Here's how the part is built. I have some questions about the finished solid (model axes, mm). A direction names the side the tool comes from. Coordinates: 2 decimals unless noted, no trailing zeros. Loops run counter-clockwise (first coordinate to the right, second up) from the corner with the lowest first, then second, coordinate; pieces in that order, holes last. Notation, with made-up numbers: (14.5, 75) -> (46.5, 75) arc R11 ccw to (46.5, 91) -> close; hole circle Ø8 at (-1, 76.25). An arc over 180 degrees is marked (long way). Answer as a JSON object with one key per item and string values. Group by question number.
Q1. I want a section at C-C on y = -27. Write out the boundary of the cut face in (x, z), then the cut area to 3 significant figures.
Q2. I need wall thicknesses on line 1 (Y direction, x = -29, z = 10); line 2 (X direction, y = -6, z = 9); line 3 (Y direction, x = -20.5, z = 7.5). Which ranges of each line are inside material? Lowest first, please.
Q3. I want a section at A-A on z = 9.5. Count the separate pieces of the cut face and the enclosed holes in it, then the cut area to 3 significant figures.
Q4. I'm going to push flat-ended pins straight in: pin 1 (6 mm diameter, centred on x = -12, y = -9, fed in from -Z); pin 2 (8.5 mm diameter, centred on x = 16.84, y = 10.22, fed in from +Z). Where does each tip first touch, or does it pass through?
Q5. On a 3-axis mill with a long thin cutter (end or side, diameter ignored), from which of +Z, -Z, +X, -X, +Y, -Y can I reach the whole of each face in a straight line? I mean faces 1 (the flat face through (2, 39.573, 6)), 2 (the cylindrical face through (-32.5, 19.4, 9.6)). Say none if no direction works.
Q6. I want a section at D-D on x = -29. Write out the boundary of the cut face in (y, z), then the cut area to 3 significant figures.
Q7. I want a section at B-B on x = 0. Write out the boundary of the cut face in (y, z).
Q8. Thinking about a two-plate mould opening in X: for faces 3 (the flat face through (41.3, -8, 6)), 4 (the cylindrical face through (-30.02, -5.32, 9.57)), 5 (the flat face through (-1, -53.676, 6)), 6 (the flat face through (17, 10, 6.35)), which applies, released by +X, released by -X, zero draft, split by the parting line, or undercut?
```python
from build123d import *

# Parameters (mm, degrees)
F0_R     = 9.227752
F0_R_2   = 10.316944
F1_DEPTH = 12.7
F2_R     = 7.603738
F2_R_2   = 5.536052
F2_R_3   = 7.326338
F2_R_4   = 7.055645
F2_R_5   = 10.428743
F2_R_6   = 6.147535
F2_R_7   = 6.569287
F2_R_8   = 5.291244
F3_DEPTH = 6.35


with BuildPart() as f1:
    # F0 (on Top) → F1 (new body)
    with BuildSketch(Plane.XY):
        with BuildLine():
            Line((12.50172, 39.573293), (-25.80679, 39.573293))
            ThreePointArc((-25.80679, 39.573293), (-19.351501, 17.287133), (-42.451348, 15.109803))
            Line((-42.451348, 15.109803), (-42.451348, -53.675774))
            Line((-42.451348, -53.675774), (-26.046417, -53.675774))
            ThreePointArc((-26.046417, -53.675774), (-15.397607, -31.799477), (-4.748798, -53.675774))
            Line((-4.748798, -53.675774), (16.548831, -53.675774))
            Line((16.548831, -53.675774), (41.300125, -53.675774))
            Line((41.300125, -53.675774), (41.300125, -43.841226))
            ThreePointArc((41.300125, -43.841226), (32.662888, -31.226924), (41.300125, -18.612622))
            Line((41.300125, -18.612622), (41.300125, 39.573293))
            Line((41.300125, 39.573293), (31.532556, 39.573293))
            ThreePointArc((31.532556, 39.573293), (22.017138, 5.274796), (12.50172, 39.573293))
        make_face()
        with BuildLine():
            ThreePointArc((25.758617, -44.465989), (23.061133, -50.978291), (16.548831, -53.675774))
            ThreePointArc((16.548831, -53.675774), (10.036529, -37.953687), (25.758617, -44.465989))
        make_face(mode=Mode.SUBTRACT)
        with Locations((20.865915, -13.382968)):
            Circle(F0_R, mode=Mode.SUBTRACT)
        with Locations((-28.06106, -5.612212)):
            Circle(F0_R_2, mode=Mode.SUBTRACT)
        with BuildLine():
            Line((31.532556, 39.573293), (12.50172, 39.573293))
            ThreePointArc((12.50172, 39.573293), (22.017138, 5.274796), (31.532556, 39.573293))
        make_face()
        with BuildLine():
            Line((-25.80679, 39.573293), (-37.798287, 39.573293))
            ThreePointArc((-37.798287, 39.573293), (-40.274021, 38.209652), (-42.451348, 36.407427))
            Line((-42.451348, 36.407427), (-42.451348, 15.109803))
            ThreePointArc((-42.451348, 15.109803), (-19.351501, 17.287133), (-25.80679, 39.573293))
        make_face()
        with BuildLine():
            ThreePointArc((-4.748798, -53.675774), (-15.397607, -31.799477), (-26.046417, -53.675774))
            Line((-26.046417, -53.675774), (-4.748798, -53.675774))
        make_face()
        with Locations((-28.06106, -5.612212)):
            Circle(F0_R_2)
        with Locations((20.865915, -13.382968)):
            Circle(F0_R)
        with BuildLine():
            ThreePointArc((25.758617, -44.465989), (10.036529, -37.953687), (16.548831, -53.675774))
            ThreePointArc((16.548831, -53.675774), (23.061133, -50.978291), (25.758617, -44.465989))
        make_face()
        with BuildLine():
            Line((41.300125, -43.841226), (41.300125, -18.612622))
            ThreePointArc((41.300125, -18.612622), (32.662888, -31.226924), (41.300125, -43.841226))
        make_face()
    extrude(amount=F1_DEPTH)

    # F2 (on face) → F3 (cut)
    with BuildSketch(Plane.XY.offset(12.7)):
        with Locations((-26.909837, 14.246385)):
            Circle(F2_R)
        with Locations((31.802539, -24.895199)):
            Circle(F2_R_2)
        with Locations((-32.090344, -37.558652)):
            Circle(F2_R_3)
        with Locations((16.836636, 10.217104)):
            Circle(F2_R_4)
        with Locations((3.309769, -40.724512)):
            Circle(F2_R_5)
        with Locations((0, 26.046421)):
            Circle(F2_R_6)
        with Locations((-23.456169, -5.612212)):
            Circle(F2_R_7)
        with Locations((15.109802, -9.929299)):
            Circle(F2_R_8)
    extrude(amount=-F3_DEPTH, mode=Mode.SUBTRACT)


solid = f1.part
```
Result set:
{
 "1": {"outline": "(-42.45, 0) -> (41.3, 0) -> (41.3, 12.7) -> (36.92, 12.7) -> (36.92, 6.35) -> (26.68, 6.35) -> (26.68, 12.7) -> (-42.45, 12.7) -> close", "area": "999 mm²"},
 "2": {"line 1": "y = -53.68 to -44.2, -30.92 to -9.14, -2.09 to 6.94, 21.56 to 39.57", "line 2": "x = -42.45 to -30.01, -16.9 to 11.57, 18.65 to 41.3", "line 3": "y = -53.68 to -11.48, 0.25 to 10.16, 18.34 to 39.57"},
 "3": {"separate pieces": "1", "enclosed holes": "8", "area": "6,520 mm²"},
 "4": {"pin 1": "stops at z = 0", "pin 2": "stops at z = 6.35"},
 "5": {"face 1": "+Z, -Z, +X, -X, +Y", "face 2": "+Z"},
 "6": {"outline": "(-53.68, 0) -> (39.57, 0) -> (39.57, 12.7) -> (21.56, 12.7) -> (21.56, 6.35) -> (6.94, 6.35) -> (6.94, 12.7) -> (-2.09, 12.7) -> (-2.09, 6.35) -> (-9.14, 6.35) -> (-9.14, 12.7) -> (-30.92, 12.7) -> (-30.92, 6.35) -> (-44.2, 6.35) -> (-44.2, 12.7) -> (-53.68, 12.7) -> close", "area": "962 mm²"},
 "7": {"outline": "(-53.68, 0) -> (39.57, 0) -> (39.57, 12.7) -> (32.19, 12.7) -> (32.19, 6.35) -> (19.9, 6.35) -> (19.9, 12.7) -> (-30.83, 12.7) -> (-30.83, 6.35) -> (-50.61, 6.35) -> (-50.61, 12.7) -> (-53.68, 12.7) -> close"},
 "8": {"face 3": "released by +X", "face 4": "undercut", "face 5": "zero draft", "face 6": "undercut"}
}
